Check sheet for the modelled part. Datum: model origin and axes. Units: mm. Face numbers are marked on the shaded views. A direction names the side the tool comes from. Coordinates: 2 decimals unless noted, no trailing zeros. Write each loop counter-clockwise with the first axis right and the second up, starting at its lowest first coordinate (ties: lowest second). Pieces come first, ordered by that corner, then holes. Notation, with made-up numbers: (-37, 73) - (-5, 73) arc R33 ccw to (-5, 107) - close; hole circle Ø7 at (1, 74). An arc over 180 degrees is marked (long way). Use one line per item in the form item = value. Start each with the question number.
1. Scan lines: line 1 along X through (y, z) = (31, -4.75); line 2 along Y through (x, z) = (51.5, -5.75); line 3 along Z through (x, y) = (32.5, 4). Record each from-to range of solid material in increasing order.
2. Draft check along Y on the marked faces 3, 4 and 5. Enter one of: +Y half, -Y half, draft (parallel to the pull), parting line (faces both ways), or undercut.
3. Tool access check on the marked faces 1 and 2. Record the directions out of +Z, -Z, +X, -X, +Y, -Y that give a thin tool (end or side, any length) a straight path to the whole face; none if there is none.
4. Cross-section at C-C on z = -3.75. Record the boundary of the cut face in (x, y).
5. Cross-section at D-D on y = 6. Record the boundary of the cut face in (x, z).
6. Cross-section at A-A on x = 55. Record the boundary of the cut face in (y, z), then the cut area to 3 significant figures.
7. Cross-section at B-B on y = 18.5. Record the boundary of the cut face in (x, z), then the cut area to 3 significant figures.
8. Go/stop test with flat-tipped pins: pin 1 Ø4 at (x, y) = (40, 16.5) entering from -Z; pin 2 Ø4 at (y, z) = (20, -4.5) entering from -X; pin 3 Ø3 at (x, z) = (34, -2.5) entering from +Y. Record where each tip stops, or that it passes through.
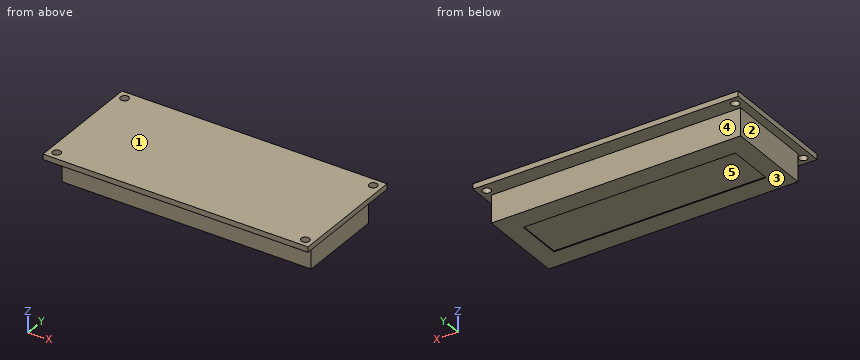
```python
from build123d import *

# Parameters (mm, degrees)
SKETCH1_W           = 80.01
SKETCH1_H           = 35.9918
BOSS_EXTRUDE1_DEPTH = 1.6002
SKETCH1_3_W         = 75.2094
SKETCH1_3_H         = 26.1874
BOSS_EXTRUDE2_DEPTH = 8.3058
SKETCH2_W           = 64.008
SKETCH2_H           = 13.9954
CUT_EXTRUDE1_DEPTH  = 0.254
SKETCH3_R           = 1.2446
CUT_EXTRUDE2_DEPTH  = 2.54


with BuildPart() as part:
    # Sketch1 → Boss-Extrude1 (new body)
    with BuildSketch(Plane.XY):
        with Locations((40.005, 17.9959)):
            Rectangle(SKETCH1_W, SKETCH1_H)
    extrude(amount=BOSS_EXTRUDE1_DEPTH)

    # Sketch1<3> → Boss-Extrude2 (add)
    with BuildSketch(Plane.XY):
        with Locations((40.0939, 17.9959)):
            Rectangle(SKETCH1_3_W, SKETCH1_3_H)
    extrude(amount=-BOSS_EXTRUDE2_DEPTH)

    # Sketch2 → Cut-Extrude1 (cut)
    with BuildSketch(Plane(origin=(0, 0, -8.3058), x_dir=(-1, 0, 0), z_dir=(0, 0, -1))):
        with Locations((-40.0939, 17.9959)):
            Rectangle(SKETCH2_W, SKETCH2_H)
    extrude(amount=-CUT_EXTRUDE1_DEPTH, mode=Mode.SUBTRACT)

    # Sketch3 → Cut-Extrude2 (cut)
    with BuildSketch(Plane(origin=(0, 0, 0), x_dir=(-1, 0, 0), z_dir=(0, 0, -1))):
        with Locations((-77.5208, 2.4892)):
            Circle(SKETCH3_R)
        with Locations((-77.5208, 33.5026)):
            Circle(SKETCH3_R)
        with Locations((-2.4892, 33.5026)):
            Circle(SKETCH3_R)
        with Locations((-2.4892, 2.4892)):
            Circle(SKETCH3_R)
    extrude(amount=-CUT_EXTRUDE2_DEPTH, mode=Mode.SUBTRACT)


solid = part.part
```
Final values:
q1.line_1 = 2.49 to 77.7
q1.line_2 = 4.9 to 31.09
q1.line_3 = 0 to 1.6
q2.face_3 = draft
q2.face_4 = +Y half
q2.face_5 = undercut
q3.face_1 = +Z, +X, -X, +Y, -Y
q3.face_2 = -Z, -X, +Y, -Y
q4.outline = (2.49, 4.9) - (77.7, 4.9) - (77.7, 31.09) - (2.49, 31.09) - close
q5.outline = (0, 0) - (2.49, 0) - (2.49, -8.31) - (77.7, -8.31) - (77.7, 0) - (80.01, 0) - (80.01, 1.6) - (0, 1.6) - close
q6.outline = (0, 0) - (4.9, 0) - (4.9, -8.31) - (11, -8.31) - (11, -8.05) - (24.99, -8.05) - (24.99, -8.31) - (31.09, -8.31) - (31.09, 0) - (35.99, 0) - (35.99, 1.6) - (0, 1.6) - close
q6.area = 272 mm²
q7.outline = (0, 0) - (2.49, 0) - (2.49, -8.31) - (8.09, -8.31) - (8.09, -8.05) - (72.1, -8.05) - (72.1, -8.31) - (77.7, -8.31) - (77.7, 0) - (80.01, 0) - (80.01, 1.6) - (0, 1.6) - close
q7.area = 736 mm²
q8.pin_1 = -8.05
q8.pin_2 = 2.49
q8.pin_3 = 31.09
